from build123d import *

# Parameters (mm, degrees)
ESQUISSE1_R        = 17.5
BOSS_EXTRU_1_DEPTH = 100
CONG_1_R           = 17
ESQUISSE2_R        = 2
BOSS_EXTRU_2_DEPTH = 25


with BuildPart() as part:
    # Esquisse1 → Boss.-Extru.1 (new body)
    with BuildSketch(Plane.XY):
        Circle(ESQUISSE1_R)
    extrude(amount=BOSS_EXTRU_1_DEPTH)

    # Congé1
    cong_1_edges = [part.edges().sort_by_distance(p)[0] for p in [
        (-17.5, 0, 0),
    ]]
    fillet(cong_1_edges, radius=CONG_1_R)

    # Esquisse2 → Boss.-Extru.2 (add)
    with BuildSketch(Plane.XY.offset(100)):
        Circle(ESQUISSE2_R)
    extrude(amount=BOSS_EXTRU_2_DEPTH)


solid = part.part
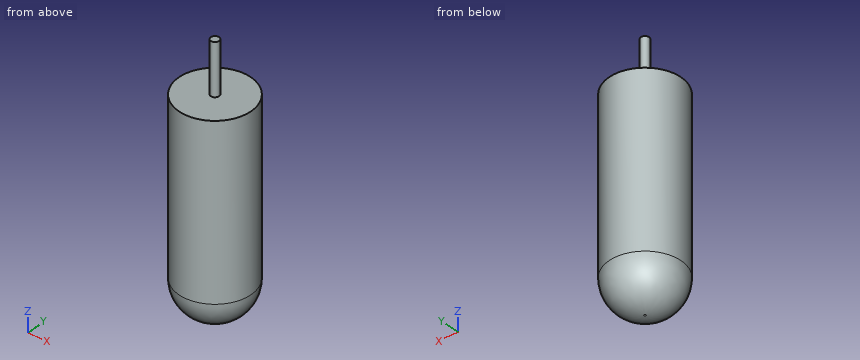
Part model, mm, in its own coordinate system. Coordinates: 2 decimals unless noted, no trailing zeros. Order: outer loops, then holes, each group sorted by start corner. A loop starts at its lowest first (then second) coordinate and runs counter-clockwise, first axis right, second up. Notation, with made-up numbers: M 87.25,-22 L 126.25,-22 A21 cw 126.25,-2 Z; hole C 32,26 d10. An arc over 180 degrees is marked long. One line per question, with ' | ' between items.
Q1. Slice it at A-A (z = 68). Give the cut face in (x, y), and give its area (3 significant figures).
A:
outline: C 0,0 d35 | area: 962 mm^2
Q2. Slice it at B-B (z = 109). Give the cut face in (x, y), and give its area (3 significant figures).
A:
outline: C 0,0 d4 | area: 12.6 mm^2
Q3. Drill centre lines: line 1 (Y direction, x = -5.5, z = 86); line 2 (X direction, y = -10, z = 18); line 3 (X direction, y = -12, z = 8). Where is each one in solid material? Low to high.
A:
line 1: y = -16.61 to 16.61 | line 2: x = -14.36 to 14.36 | line 3: x = -8.87 to 8.87
Q4. Pin check, flat tips, straight feed: P1, Ø1, axis at y = 12.5, z = 77.5, coming from the +X side; P2, Ø2, axis at x = 8, y = -13.5, coming from the +Z side; P3, Ø1.5, axis at y = 2.5, z = 65, coming from the -X side. Stop position of each tip, or through.
A:
P1: stops at x = 12.74 | P2: stops at z = 100 | P3: stops at x = -17.41
